from build123d import *

# Parameters (mm, degrees)
F1_DEPTH = 20.0152
F3_DEPTH = 15
F4_R     = 2.75
F5_DEPTH = 19.7838
F8_DEPTH = 4


with BuildPart() as f1:
    # F0 (on Top) → F1 (new body)
    with BuildSketch(Plane.XY):
        with BuildLine():
            ThreePointArc((-81, 3), (-85, -5), (-89, 3))
            Line((-89, 3), (-89, 5))
            Line((-89, 5), (-89.8989794856, 5))
            ThreePointArc((-89.8989794856, 5), (-91.9953543967, 0.2549840475), (-90.25, -4.6300647944))
            ThreePointArc((-90.25, -4.6300647944), (-90.0004908056, -5.3228294538), (-90.2928932188, -5.9986094033))
            Line((-90.2928932188, -5.9986094033), (-95.0770838155, -10.7828))
            Line((-95.0770838155, -10.7828), (-106.526, -10.7828))
            Line((-106.526, -10.7828), (-106.526, -14.7828))
            Line((-106.526, -14.7828), (106.526, -14.7828))
            Line((106.526, -14.7828), (106.526, -10.7828))
            Line((106.526, -10.7828), (95.0770838155, -10.7828))
            Line((95.0770838155, -10.7828), (90.2928932188, -5.9986094033))
            ThreePointArc((90.2928932188, -5.9986094033), (90.0004908056, -5.3228294538), (90.25, -4.6300647944))
            ThreePointArc((90.25, -4.6300647944), (91.9953543967, 0.2549840475), (89.8989794856, 5))
            Line((89.8989794856, 5), (89, 5))
            Line((89, 5), (89, 3))
            ThreePointArc((89, 3), (85, -5), (81, 3))
            Line((81, 3), (81, 5))
            Line((81, 5), (80.1010205144, 5))
            ThreePointArc((80.1010205144, 5), (78.0046456033, 0.2549840475), (79.75, -4.6300647944))
            ThreePointArc((79.75, -4.6300647944), (79.9995091944, -5.3228294538), (79.7071067812, -5.9986094033))
            Line((79.7071067812, -5.9986094033), (74.9229161845, -10.7828))
            Line((74.9229161845, -10.7828), (-74.9229161845, -10.7828))
            Line((-74.9229161845, -10.7828), (-79.7071067812, -5.9986094033))
            ThreePointArc((-79.7071067812, -5.9986094033), (-79.9995091944, -5.3228294538), (-79.75, -4.6300647944))
            ThreePointArc((-79.75, -4.6300647944), (-78.0046456033, 0.2549840475), (-80.1010205144, 5))
            Line((-80.1010205144, 5), (-81, 5))
            Line((-81, 5), (-81, 3))
        make_face()
    extrude(amount=F1_DEPTH)

    # F2 (on face) → F3 (join)
    with BuildSketch(Plane.XY.offset(20.0152)):
        with BuildLine():
            Line((-89, 5), (-89.8989794856, 5))
            ThreePointArc((-89.8989794856, 5), (-91.9953543967, 0.2549840475), (-90.25, -4.6300647944))
            ThreePointArc((-90.25, -4.6300647944), (-85, -7), (-79.75, -4.6300647944))
            ThreePointArc((-79.75, -4.6300647944), (-78.0046456033, 0.2549840475), (-80.1010205144, 5))
            Line((-80.1010205144, 5), (-81, 5))
            Line((-81, 5), (-81, 3))
            ThreePointArc((-81, 3), (-85, -5), (-89, 3))
            Line((-89, 3), (-89, 5))
        make_face()
        with BuildLine():
            ThreePointArc((80.1010205144, 5), (78.0046456033, 0.2549840475), (79.75, -4.6300647944))
            ThreePointArc((79.75, -4.6300647944), (85, -7), (90.25, -4.6300647944))
            ThreePointArc((90.25, -4.6300647944), (91.9953543967, 0.2549840475), (89.8989794856, 5))
            Line((89.8989794856, 5), (89, 5))
            Line((89, 5), (89, 3))
            ThreePointArc((89, 3), (85, -5), (81, 3))
            Line((81, 3), (81, 5))
            Line((81, 5), (80.1010205144, 5))
        make_face()
    extrude(amount=F3_DEPTH)

    # F4 (on face) → F5 (cut, through all)
    with BuildSketch(Plane.XZ.offset(14.7828)):
        with Locations((-100.8270838155, 10.0076)):
            Circle(F4_R)
        with Locations((-69.1729161845, 10.0076)):
            Circle(F4_R)
        with Locations((69.1729161845, 10.0076)):
            Circle(F4_R)
        with Locations((100.8270838155, 10.0076)):
            Circle(F4_R)
    extrude(amount=-F5_DEPTH, mode=Mode.SUBTRACT)

    # F7 (on offset) → F8 (join)
    with BuildSketch(Plane.YZ.offset(-87)):
        Polygon((-7, 35.0152), (-14.7828, 20.0152), (-6, 20.0152), (-6, 35.0152), align=None)
    extrude(amount=F8_DEPTH)

    # F9: F1 across plane


with BuildPart() as f1_1:
    add(f1.part)
    add(f1.part.mirror(Plane.YZ))


solid = f1_1.part
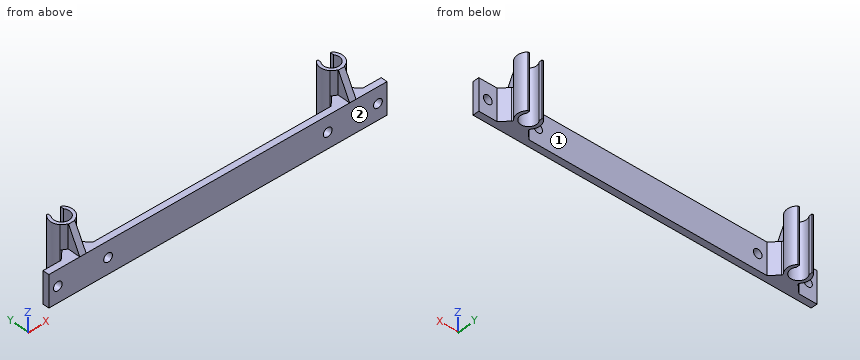
Verification items for the finished model (mm, model axes). Face numbers are marked on the shaded views. Coordinates: 2 decimals unless noted, no trailing zeros. Order: outer loops, then holes, each group sorted by start corner. A loop starts at its lowest first (then second) coordinate and runs counter-clockwise, first axis right, second up. Notation, with made-up numbers: (45, -0.75) -> (58, -0.75) arc R6 cw to (58, 7.25) -> close; hole circle Ø7 at (84, -11). An arc over 180 degrees is marked (long way). Put each result on its own line as item: value. Start each with the question number.
1. Cross-section at D-D, the plane x = -9.5. Record the boundary of the cut face in (y, z), then the cut area to 3 significant figures.
2. Cross-section at B-B, the plane x = 85. Record the boundary of the cut face in (y, z).
3. Go/stop test with flat-tipped pins: pin 1 Ø8 at (x, y) = (-93.5, -9.5) entering from +Z; pin 2 Ø9 at (x, y) = (-85, 0) entering from -Z; pin 3 Ø9 at (x, z) = (103.5, 13) entering from +Y; pin 4 Ø2.5 at (y, z) = (-11, 29.5) entering from -X. Record where each tip stops, or that it passes through.
4. Mould release check, pull along X, two halves, no side actions. Record for the marked faces 1 and 2: released by +X, released by -X, zero draft, split by the parting line, or undercut.
5. Material ranges on L1, parallel to X at y = 0, z = 10; L2, parallel to X at y = -7, z = 33; L3, parallel to X at y = -6, z = 16, recorded low to high. Write a range as [from, to].
Computed:
1. outline: (-14.78, 0) -> (-10.78, 0) -> (-10.78, 20.02) -> (-14.78, 20.02) -> close
1. area: 80.1 mm2
2. outline: (-14.78, 0) -> (-5, 0) -> (-5, 35.02) -> (-7, 35.02) -> (-14.78, 20.02) -> close
3. pin 1: z = 20.02
3. pin 2: through
3. pin 3: y = -10.78
3. pin 4: x = -87
4. face 1: undercut
4. face 2: zero draft
5. L1: [-92, -90], [-80, -78], [78, 80], [90, 92]
5. L2: [-87, -83], [83, 87]
5. L3: [-90.29, -79.71], [79.71, 90.29]
